Geometry: final body of the model. Coordinates: model frame, mm. Coordinates: 2 decimals unless noted, no trailing zeros. Order: outer loops, then holes, each group sorted by start corner. A loop starts at its lowest first (then second) coordinate and runs counter-clockwise, first axis right, second up. Notation, with made-up numbers: M 72,-24.75 L 124,-24.75 A30 cw 124,12.25 Z; hole C 85,16 d7. An arc over 180 degrees is marked long. Use CSV: the item, a comma, the result in double quotes. Start each with the question number.
1. Section query D-D on x = 0. Return the cut outline in (y, z).
2. Section query A-A on y = 1. Return the cut outline in (x, z), and give its area (3 significant figures).
3. Section query B-B on z = 6.5. Return the cut outline in (x, y).
4. Pull-direction query (X, two-part tool) for faces 1 (the flat face through (7.2, -1, 5)), 2 (the cylindrical face through (-0.1, 6.2, 5.1)), 3 (the cylindrical face through (-0.1, 5.2, 5.1)); classes: pulls with the +X half, pulls with the -X half, needs draft (parallel to the pull), parting line crosses it, or undercut.
5. Section query C-C on y = 0. Return the cut outline in (x, z).
6. First-contact query: P1, Ø1, axis at x = -3, y = 2, coming from the +Z side; P2, Ø1, axis at y = 5, z = 2, coming from the -X side (3 decimals); P3, Ø1, axis at x = 2, z = 4, coming from the -Y side; P4, Ø0.8, axis at x = -7, z = 3.5, coming from the +Y side. Flat tips, straight axial feed; report the tip coordinate or a pass-through.
7. Material intervals for line 1 (X direction, y = 0, z = 7.75); line 2 (Y direction, x = 0, z = 6.25); line 3 (X direction, y = 5.5, z = 6), sorted ascending.
Autodesk Inventor part; units mm, degrees
ref_plane "YZ Plane" through (0, 0, 0) normal (1, 0, 0) x (0, 1, 0)
ref_plane "XZ Plane" through (0, 0, 0) normal (0, 1, 0) x (-1, 0, 0)
ref_plane "XY Plane" through (0, 0, 0) normal (0, 0, 1) x (1, 0, 0)
sketch "스케치1" plane through (0, 0, 0) normal (0, 0, 1) x (1, 0, 0)
  arc A0 (4.9143, -1.7) -> (-4.9143, -1.7) centre (0, 0) ccw
  line L0 (-7.2, -1.7) -> (-7.2, -0.7)
  line L1 (7.2, -0.7) -> (7.2, -1.7)
  arc A1 (5.9624, -1.7) -> (-6.1604, -0.7) centre (0, 0) ccw
  line L2 (-7.2, -1.7) -> (-4.9143, -1.7)
  line L3 (4.9143, -1.7) -> (7.2, -1.7)
  line L4 (-7.2, -0.7) -> (-5.1527, -0.7)
  line L5 (5.1527, -0.7) -> (7.2, -0.7)
  point P0 (0, -0.7)
  point P1 (6.1604, -0.7)
  dimension "d0" = 10.4
  dimension "d1" = 1
  dimension "d2" = 0.7
  dimension "d3" = 2
  dimension "d4" = 1
extrude "돌출1" add sketch "스케치1" along normal blind 10.4
properties part number "rotion_stopper"
Results list:
1,outline,"M 5.2,0 L 6.2,0 L 6.2,10.4 L 5.2,10.4 Z"
2,outline,"M -6.12,0 L -5.1,0 L -5.1,10.4 L -6.12,10.4 Z; M 5.1,0 L 6.12,0 L 6.12,10.4 L 5.1,10.4 Z"
2,area,"21.1 mm²"
3,outline,"M -7.2,-1.7 L -4.91,-1.7 A5.2 cw long 4.91,-1.7 L 7.2,-1.7 L 7.2,-0.7 L 6.16,-0.7 A6.2 ccw long -6.16,-0.7 L -7.2,-0.7 Z"
4,face 1,"pulls with the +X half"
4,face 2,"parting line crosses it"
4,face 3,"undercut"
5,outline,"M -6.2,0 L -5.2,0 L -5.2,10.4 L -6.2,10.4 Z; M 5.2,0 L 6.2,0 L 6.2,10.4 L 5.2,10.4 Z"
6,P1,"passes through"
6,P2,"stops at x = -4.265"
6,P3,"stops at y = 4.56"
6,P4,"stops at y = -0.7"
7,line 1,"x = -6.2 to -5.2, 5.2 to 6.2"
7,line 2,"y = 5.2 to 6.2"
7,line 3,"x = -2.86 to 2.86"
